```python
from build123d import *

# Parameters (mm, degrees)
SKETCH_1_R      = 1.525
SKETCH_1_W      = 16.514718626
SKETCH_1_H      = 15
EXTRUDE_1_DEPTH = 2
FILLET_1_R      = 1.5


with BuildPart() as part:
    # 草图1 → 凸台-拉伸1 (new body)
    with BuildSketch(Plane.XY):
        with BuildLine():
            Line((-8.257359313, 12.5), (8.257359313, 12.5))
            Line((8.257359313, 12.5), (13.128679656, 17.371320344))
            ThreePointArc((13.128679656, 17.371320344), (17.371320344, 17.371320344), (17.371320344, 13.128679656))
            Line((17.371320344, 13.128679656), (12.5, 8.257359313))
            Line((12.5, 8.257359313), (12.5, -8.257359313))
            Line((12.5, -8.257359313), (17.371320344, -13.128679656))
            ThreePointArc((17.371320344, -13.128679656), (17.371320344, -17.371320344), (13.128679656, -17.371320344))
            Line((13.128679656, -17.371320344), (8.257359313, -12.5))
            Line((8.257359313, -12.5), (-8.257359313, -12.5))
            Line((-8.257359313, -12.5), (-13.128679656, -17.371320344))
            ThreePointArc((-13.128679656, -17.371320344), (-17.371320344, -17.371320344), (-17.371320344, -13.128679656))
            Line((-17.371320344, -13.128679656), (-12.5, -8.257359313))
            Line((-12.5, -8.257359313), (-12.5, 8.257359313))
            Line((-12.5, 8.257359313), (-17.371320344, 13.128679656))
            ThreePointArc((-17.371320344, 13.128679656), (-17.371320344, 17.371320344), (-13.128679656, 17.371320344))
            Line((-13.128679656, 17.371320344), (-8.257359313, 12.5))
        make_face()
        with Locations((-15.25, 15.25)):
            Circle(SKETCH_1_R, mode=Mode.SUBTRACT)
        with Locations((15.25, 15.25)):
            Circle(SKETCH_1_R, mode=Mode.SUBTRACT)
        with Locations((-15.25, -15.25)):
            Circle(SKETCH_1_R, mode=Mode.SUBTRACT)
        with Locations((15.25, -15.25)):
            Circle(SKETCH_1_R, mode=Mode.SUBTRACT)
        with Locations((-10, 10)):
            Circle(SKETCH_1_R, mode=Mode.SUBTRACT)
        with Locations(Location((10, 10, 0), (0, 0, 180))):
            Circle(SKETCH_1_R, mode=Mode.SUBTRACT)
        with Locations((10, -10)):
            Circle(SKETCH_1_R, mode=Mode.SUBTRACT)
        with Locations(Location((-10, -10, 0), (0, 0, 180))):
            Circle(SKETCH_1_R, mode=Mode.SUBTRACT)
        Rectangle(SKETCH_1_W, SKETCH_1_H, mode=Mode.SUBTRACT)
    extrude(amount=EXTRUDE_1_DEPTH)

    # 圆角1
    fillet_1_edges = [part.edges().sort_by_distance(p)[0] for p in [
        (-8.257359313, 12.5, 1),
        (8.257359313, 12.5, 1),
        (12.5, 8.257359313, 1),
        (12.5, -8.257359313, 1),
        (8.257359313, -12.5, 1),
        (-8.257359313, -12.5, 1),
        (-12.5, -8.257359313, 1),
        (-12.5, 8.257359313, 1),
        (-8.257359313, 7.5, 1),
        (-8.257359313, -7.5, 1),
        (8.257359313, -7.5, 1),
        (8.257359313, 7.5, 1),
    ]]
    fillet(fillet_1_edges, radius=FILLET_1_R)


solid = part.part
```
Build history of the part. All positions in model axes, mm. A direction names the side the tool comes from. Give positions to 0.01 mm unless a question says otherwise; leave off trailing zeros. Loops run counter-clockwise (first coordinate to the right, second up) from the corner with the lowest first, then second, coordinate; pieces in that order, holes last.
1) Drop flat-ended pins along their axis: P1, Ø1, axis at y = -3.5, z = 1, coming from the -X side; P2, Ø1, axis at y = -3, z = 0.5, coming from the +X side; P3, Ø0.6, axis at x = 2, z = 1.5, coming from the +Y side. Give the stop position or say it passes through.
Values follow:
P1: stops at x = -12.5
P2: stops at x = 12.5
P3: stops at y = 12.5
2) Two-plate mould, pull along X, no slides. Class faces 4 (the face through (0, 8, 2)), 5 (the face through (15.12, -10.88, 0.99)), 6 (the face through (-7.83, 7.05, 1.01)): released by +X, released by -X, zero draft, split by the parting line, or undercut.
Values follow:
face 4: zero draft
face 5: released by +X
face 6: undercut
3) 3-axis set-ups, long thin cutter, end or side, ignore diameter. For faces 1 (the face through (-10.88, -15.12, 0.99)), 2 (the face through (-10.944, 15.186, 0.986)), 3 (the face through (-12.62, 8.22, 1.01)): which of +Z, -Z, +X, -X, +Y, -Y reach the whole face in a straight line?
Values follow:
face 1: +Z, -Z, -Y
face 2: +Z, -Z, +Y
face 3: +Z, -Z, -X
4) Band-saw the part on B-B on x = -10. List the corners of the cut face in (y, z) (3 decimals).
Values follow:
outline: (-14.243, 0) - (-11.525, 0) - (-11.525, 2) - (-14.243, 2) - close; (-8.475, 0) - (8.475, 0) - (8.475, 2) - (-8.475, 2) - close; (11.525, 0) - (14.243, 0) - (14.243, 2) - (11.525, 2) - close
5) Band-saw the part on C-C on x = 15.25. List the corners of the cut face in (y, z) (3 decimals).
Values follow:
outline: (-18.25, 0) - (-16.775, 0) - (-16.775, 2) - (-18.25, 2) - close; (-13.725, 0) - (-11.007, 0) - (-11.007, 2) - (-13.725, 2) - close; (11.007, 0) - (13.725, 0) - (13.725, 2) - (11.007, 2) - close; (16.775, 0) - (18.25, 0) - (18.25, 2) - (16.775, 2) - close
6) Band-saw the part on A-A on y = -1.5. List the corners of the cut face in (x, z), then the cut area to 3 significant figures.
Values follow:
outline: (-12.5, 0) - (-8.26, 0) - (-8.26, 2) - (-12.5, 2) - close; (8.26, 0) - (12.5, 0) - (12.5, 2) - (8.26, 2) - close
area: 17.0 mm2
7) Probe line 1 along Y through (x, z) = (0, 1.9); line 2 along X through (y, z) = (3.5, 1.55); line 3 along Y through (x, z) = (10, 1.55) (3 decimals). List the from-to ranges inside material, lowest first.
Values follow:
line 1: y = -12.5 to -7.5, 7.5 to 12.5
line 2: x = -12.5 to -8.26, 8.26 to 12.5
line 3: y = -14.243 to -11.525, -8.475 to 8.475, 11.525 to 14.243
